Verification items for the finished model (mm, model axes). Give positions to 0.01 mm unless a question says otherwise; leave off trailing zeros. Write each loop counter-clockwise with the first axis right and the second up, starting at its lowest first coordinate (ties: lowest second). Pieces come first, ordered by that corner, then holes. Notation, with made-up numbers: (-25.75, 83) -> (12.25, 83) arc R17 cw to (12.25, 87) -> close; hole circle Ø5 at (66, 58). An arc over 180 degrees is marked (long way). Answer as CSV lines item,"result".
```python
from build123d import *

# Parameters (mm, degrees)
SKETCH1_R                   = 13.5
SKETCH1_R_2                 = 9.525
F_1_4_CLEARANCE_HOLE2_D     = 6.7564
F_1_4_CLEARANCE_HOLE2_DEPTH = 13.5


with BuildPart() as part:
    # Sweep1: sweep along a curve in space
    with BuildLine() as sweep1_path:
        Line((0, 0, 0), (0, 0, -265))
    # Sketch1 → Sweep1 (sweep)
    with BuildSketch(Plane.XY):
        Circle(SKETCH1_R)
        Circle(SKETCH1_R_2, mode=Mode.SUBTRACT)
    sweep(path=sweep1_path.line)

    # 1/4 Clearance Hole2
    with Locations(Plane(origin=(13.5, 0, -215), x_dir=(0, 1, 0), z_dir=(1, 0, 0))):
        with Locations((0, 0), (0, 160), (0, 120), (0, 80), (0, 40)):
            Hole(F_1_4_CLEARANCE_HOLE2_D / 2, depth=F_1_4_CLEARANCE_HOLE2_DEPTH)


solid = part.part
```
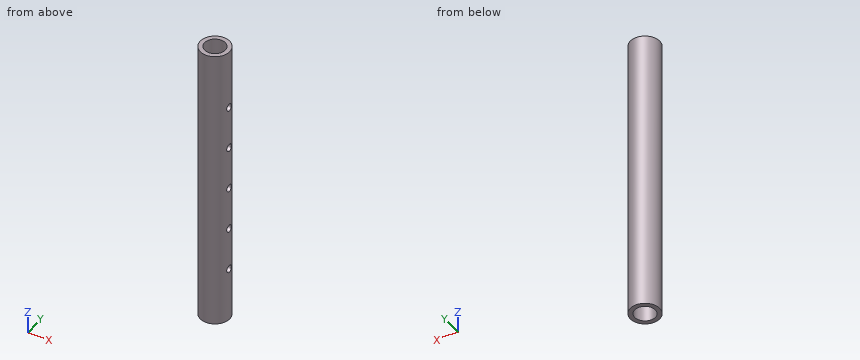
1) Depth check by flat-ended pin: pin 1 (3 mm diameter, centred on x = -4.5, z = -103.5, fed in from -Y); pin 2 (4 mm diameter, centred on x = -10.5, z = -141.5, fed in from -Y); pin 3 (10 mm diameter, centred on y = 5.5, z = -106, fed in from +X). Enter the tip coordinate at first touch or a pass-through.
Reported:
pin 1,"y = -13.16"
pin 2,"y = -10.49"
pin 3,"x = 13.49"
2) Section check A-A (x = 0). Record the boundary of the cut face in (y, z) (3 decimals).
Reported:
outline,"(-13.5, -265) -> (-9.525, -265) -> (-9.525, 0) -> (-13.5, 0) -> close; (9.525, -265) -> (13.5, -265) -> (13.5, 0) -> (9.525, 0) -> close"
3) Section check B-B (y = -6). Record the boundary of the cut face in (x, z).
Reported:
outline,"(-12.09, -265) -> (-7.4, -265) -> (-7.4, 0) -> (-12.09, 0) -> close; (7.4, -265) -> (12.09, -265) -> (12.09, 0) -> (7.4, 0) -> close"
4) Scan lines: line 1 along Z through (x, y) = (11.15, 0); line 2 along X through (y, z) = (0.5, -238); line 3 along Y through (x, z) = (0, -163.5) (3 decimals). Record each from-to range of solid material in increasing order.
Reported:
line 1,"-265 to -218.38, -211.62 to -178.38, -171.62 to -138.38, -131.62 to -98.38, -91.62 to -58.38, -51.62 to 0"
line 2,"-13.49 to -9.51, 9.51 to 13.49"
line 3,"-13.5 to -9.525, 9.525 to 13.5"
